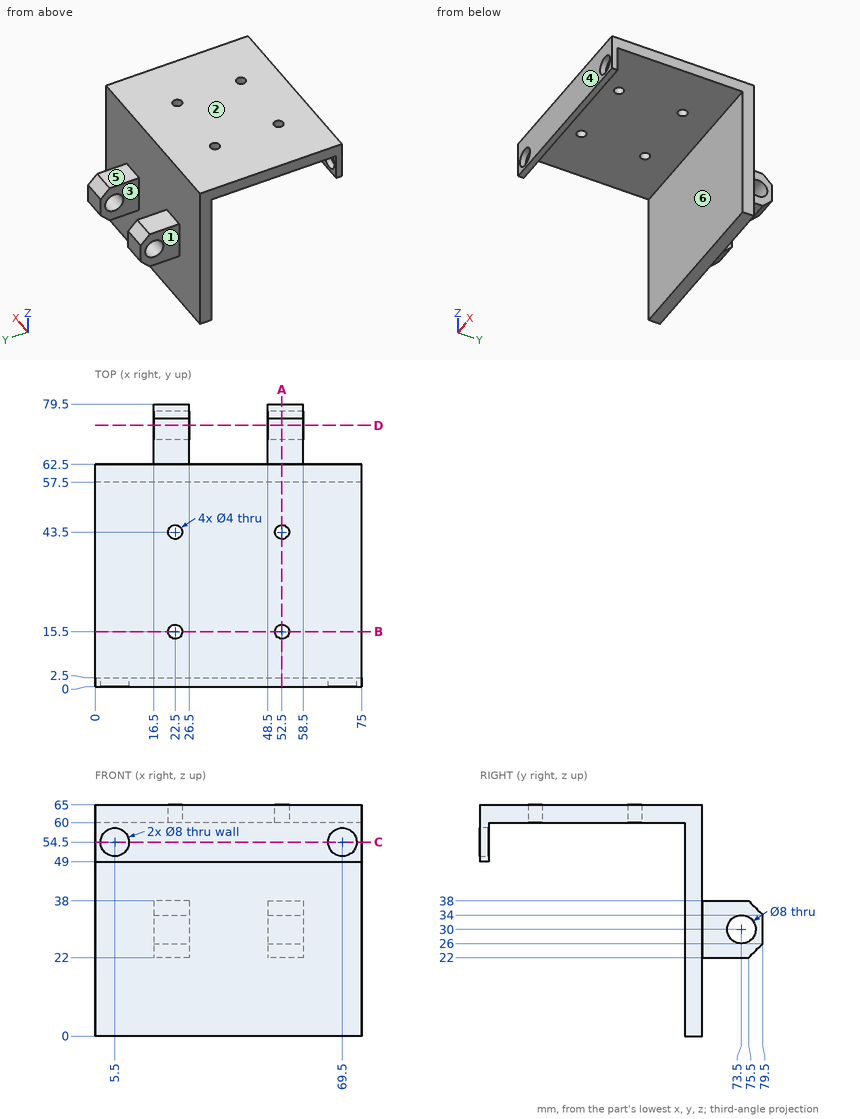
Print and shaded views of the part. All mm, measured from the part's lowest x, y and z. A direction names the side the tool comes from. Give positions to 0.01 mm unless a question says otherwise; leave off trailing zeros. Loops run counter-clockwise (first coordinate to the right, second up) from the corner with the lowest first, then second, coordinate; pieces in that order, holes last. Notation, with made-up numbers: (-24, 71.5) -> (-12, 71.5) arc R17 ccw to (-12, 96.5) -> close; hole circle Ø4 at (20, 89.25). An arc over 180 degrees is marked (long way). Answer in a Markdown table with one row per item.
Item 1: Probe line 1 along X through (y, z) = (1.3, 54.5); line 2 along Y through (x, z) = (52.5, 63.25); line 3 along Z through (x, y) = (47, 26.5). List the from-to ranges inside material, lowest first. Write a range as [from, to].
Findings below:
| item | result |
|---|---|
| line 1 | x = [0, 1.5], [9.5, 65.5], [73.5, 75] |
| line 2 | y = [0, 13.5], [17.5, 41.5], [45.5, 62.5] |
| line 3 | z = [60, 65] |
Item 2: Slice it at A-A on x = 52.5. Write the cut outline in (y, z), plus the area to 3 significant figures.
Findings below:
| item | result |
|---|---|
| outline | (0, 49) -> (2.5, 49) -> (2.5, 60) -> (13.5, 60) -> (13.5, 65) -> (0, 65) -> close; (17.5, 60) -> (41.5, 60) -> (41.5, 65) -> (17.5, 65) -> close; (45.5, 60) -> (57.5, 60) -> (57.5, 0) -> (62.5, 0) -> (62.5, 22) -> (75.5, 22) -> (79.5, 26) -> (79.5, 34) -> (75.5, 38) -> (62.5, 38) -> (62.5, 65) -> (45.5, 65) -> close; hole circle Ø8 at (73.5, 30) |
| area | 806 mm² |
Item 3: Slice it at B-B on y = 15.5. Write the cut outline in (x, z).
Findings below:
| item | result |
|---|---|
| outline | (0, 60) -> (20.5, 60) -> (20.5, 65) -> (0, 65) -> close; (24.5, 60) -> (50.5, 60) -> (50.5, 65) -> (24.5, 65) -> close; (54.5, 60) -> (75, 60) -> (75, 65) -> (54.5, 65) -> close |
Item 4: Tool access for the marked faces 4, 5 and 6: list every direction of +Z, -Z, +X, -X, +Y, -Y with a clear straight run to the whole face (end or side of a thin tool).
Findings below:
| item | result |
|---|---|
| face 4 | +Z, -Z, +X, -X, -Y |
| face 5 | +Z, +X, -X, +Y |
| face 6 | -Z, +X, -X |
Item 5: Slice it at C-C on z = 54.5. Write the cut outline in (x, y), plus the area to 4 significant figures.
Findings below:
| item | result |
|---|---|
| outline | (0, 0) -> (1.5, 0) -> (1.5, 2.5) -> (0, 2.5) -> close; (0, 57.5) -> (75, 57.5) -> (75, 62.5) -> (0, 62.5) -> close; (9.5, 0) -> (65.5, 0) -> (65.5, 2.5) -> (9.5, 2.5) -> close; (73.5, 0) -> (75, 0) -> (75, 2.5) -> (73.5, 2.5) -> close |
| area | 522.5 mm² |
Item 6: Mould opens along X. For the marked faces 1, 2 and 3 say: pulls with the +X half, pulls with the -X half, needs draft (parallel to the pull), parting line crosses it, or undercut.
Findings below:
| item | result |
|---|---|
| face 1 | pulls with the -X half |
| face 2 | needs draft |
| face 3 | undercut |
Item 7: Slice it at D-D on y = 73.5. Write the cut outline in (x, z), plus the area to 3 significant figures.
Findings below:
| item | result |
|---|---|
| outline | (16.5, 22) -> (26.5, 22) -> (26.5, 26) -> (16.5, 26) -> close; (16.5, 34) -> (26.5, 34) -> (26.5, 38) -> (16.5, 38) -> close; (48.5, 22) -> (58.5, 22) -> (58.5, 26) -> (48.5, 26) -> close; (48.5, 34) -> (58.5, 34) -> (58.5, 38) -> (48.5, 38) -> close |
| area | 160 mm² |
Item 8: Flat gauge pins, fed straight in: P1, Ø3, axis at x = 52.5, y = 43.5, coming from the +Z side; P2, Ø8, axis at y = 72.5, z = 31, coming from the -X side; P3, Ø6, axis at x = 25, z = 19, coming from the -Y side; P4, Ø11, axis at x = 55.5, y = 71, coming from the -Z side. Where does each tip first touch, or does it go through?
Findings below:
| item | result |
|---|---|
| P1 | passes through |
| P2 | stops at x = 16.5 |
| P3 | stops at y = 57.5 |
| P4 | stops at z = 22 |
